Input: part model. Units: mm. Frame: model coordinates. Round coordinates to 2 decimals unless told otherwise and drop trailing zeros. Loops run counter-clockwise (first coordinate to the right, second up) from the corner with the lowest first, then second, coordinate; pieces in that order, holes last. Notation, with made-up numbers: M -10,76 L 47,76 A16 ccw 47,89 Z; hole C 18,52 d3. An arc over 180 degrees is marked long. Use one line per item in the form item = value. Start each with the question number.
Q1. Section query C-C, the plane y = 0. State how many separate pieces and enclosed holes the cut face has, and give its area (3 significant figures).
Q2. Section query B-B, the plane z = 3. Output: boundary loops of the cut face in (x, y) (3 decimals), and give its area (3 significant figures).
Q3. Mould query, pull axis Z, two halves, no side actions, for faces 1 (the cylindrical face through (7.4, -0.04, 23.75)), 2 (the flat face through (0, 2.925, 0)), 3 (the cylindrical face through (-25.24, 0.04, -5.6)). Classes: pulls with the +Z half, pulls with the -Z half, needs draft (parallel to the pull), parting line crosses it, or undercut.
Q4. Section query A-A, the plane x = 15. Output: boundary loops of the cut face in (y, z) (3 decimals).
Q5. First-contact query: P1, Ø3, axis at y = 2, z = -5.5, coming from the +X side. Flat tip, straight axial feed; report the tip coordinate or a pass-through.
Q6. Ray query, line 1 along Z through (x, y) = (13, -0.15); line 2 along X through (y, z) = (0.25, 6); line 3 along X through (y, z) = (-2.4, -21). Return the intervals inside material, ascending.
```python
from build123d import *

# Parameters (mm, degrees)
SKETCH1_R           = 25.85370091
BOSS_EXTRUDE1_DEPTH = 2.925
CUT_EXTRUDE1_DEPTH  = 38.02769506


with BuildPart() as part:
    # Sketch1 → Boss-Extrude1 (new, symmetric)
    with BuildSketch(Plane(origin=(0, 0, 0), x_dir=(1, 0, 0), z_dir=(0, 1, 0))):
        with Locations(Location((0, 0, 0), (0, 0, 270))):
            Circle(SKETCH1_R)
    extrude(amount=BOSS_EXTRUDE1_DEPTH, both=True)

    # Sketch2 → Cut-Extrude1 (cut, through all)
    with BuildSketch(Plane.XZ.offset(2.925)):
        with BuildLine():
            ThreePointArc((22.019698731, -5.602620776), (21.872491194, -7.364247848), (23.634118266, -7.511455385))
            ThreePointArc((23.634118266, -7.511455385), (23.781325803, -5.749828313), (22.019698731, -5.602620776))
        make_face()
        with BuildLine():
            ThreePointArc((22.791373624, 3.631983723), (22.644166087, 1.87035665), (24.405793159, 1.723149114))
            ThreePointArc((24.405793159, 1.723149114), (24.553000696, 3.484776186), (22.791373624, 3.631983723))
        make_face()
        with BuildLine():
            ThreePointArc((17.772833946, -13.838975667), (17.625626409, -15.600602739), (19.387253481, -15.747810276))
            ThreePointArc((19.387253481, -15.747810276), (19.534461018, -13.986183203), (17.772833946, -13.838975667))
        make_face()
        with BuildLine():
            ThreePointArc((10.697325934, -19.82317058), (10.550118397, -21.584797652), (12.311745469, -21.732005189))
            ThreePointArc((12.311745469, -21.732005189), (12.458953006, -19.970378117), (10.697325934, -19.82317058))
        make_face()
        with BuildLine():
            ThreePointArc((1.87035665, -22.644166087), (1.723149114, -24.405793159), (3.484776186, -24.553000696))
            ThreePointArc((3.484776186, -24.553000696), (3.631983723, -22.791373624), (1.87035665, -22.644166087))
        make_face()
        with BuildLine():
            ThreePointArc((-7.364247848, -21.872491194), (-7.511455385, -23.634118266), (-5.749828313, -23.781325803))
            ThreePointArc((-5.749828313, -23.781325803), (-5.602620776, -22.019698731), (-7.364247848, -21.872491194))
        make_face()
        with BuildLine():
            ThreePointArc((-15.600602739, -17.625626409), (-15.747810276, -19.387253481), (-13.986183203, -19.534461018))
            ThreePointArc((-13.986183203, -19.534461018), (-13.838975667, -17.772833946), (-15.600602739, -17.625626409))
        make_face()
        with BuildLine():
            ThreePointArc((-21.584797652, -10.550118397), (-21.732005189, -12.311745469), (-19.970378117, -12.458953006))
            ThreePointArc((-19.970378117, -12.458953006), (-19.82317058, -10.697325934), (-21.584797652, -10.550118397))
        make_face()
        with BuildLine():
            ThreePointArc((-24.405793159, -1.723149114), (-24.553000696, -3.484776186), (-22.791373624, -3.631983723))
            ThreePointArc((-22.791373624, -3.631983723), (-22.644166087, -1.87035665), (-24.405793159, -1.723149114))
        make_face()
        with BuildLine():
            ThreePointArc((-23.634118266, 7.511455385), (-23.781325803, 5.749828313), (-22.019698731, 5.602620776))
            ThreePointArc((-22.019698731, 5.602620776), (-21.872491194, 7.364247848), (-23.634118266, 7.511455385))
        make_face()
        with BuildLine():
            ThreePointArc((-19.387253481, 15.747810276), (-19.534461018, 13.986183203), (-17.772833946, 13.838975667))
            ThreePointArc((-17.772833946, 13.838975667), (-17.625626409, 15.600602739), (-19.387253481, 15.747810276))
        make_face()
        with BuildLine():
            ThreePointArc((-12.311745469, 21.732005189), (-12.458953006, 19.970378117), (-10.697325934, 19.82317058))
            ThreePointArc((-10.697325934, 19.82317058), (-10.550118397, 21.584797652), (-12.311745469, 21.732005189))
        make_face()
        with BuildLine():
            ThreePointArc((-3.484776186, 24.553000696), (-3.631983723, 22.791373624), (-1.87035665, 22.644166087))
            ThreePointArc((-1.87035665, 22.644166087), (-1.723149114, 24.405793159), (-3.484776186, 24.553000696))
        make_face()
        with BuildLine():
            ThreePointArc((5.749828313, 23.781325803), (5.602620776, 22.019698731), (7.364247848, 21.872491194))
            ThreePointArc((7.364247848, 21.872491194), (7.511455385, 23.634118266), (5.749828313, 23.781325803))
        make_face()
        with BuildLine():
            ThreePointArc((19.970378117, 12.458953006), (19.82317058, 10.697325934), (21.584797652, 10.550118397))
            ThreePointArc((21.584797652, 10.550118397), (21.732005189, 12.311745469), (19.970378117, 12.458953006))
        make_face()
        with BuildLine():
            ThreePointArc((13.986183203, 19.534461018), (13.838975667, 17.772833946), (15.600602739, 17.625626409))
            ThreePointArc((15.600602739, 17.625626409), (15.747810276, 19.387253481), (13.986183203, 19.534461018))
        make_face()
    extrude(amount=-CUT_EXTRUDE1_DEPTH, mode=Mode.SUBTRACT)


solid = part.part
```
Results found:
q1.separate_pieces = 1
q1.enclosed_holes = 16
q1.area = 2,020 mm²
q2.outline = M -25.679,-2.925 L 22.391,-2.925 L 22.391,2.925 L -25.679,2.925 Z; M 24.806,-2.925 L 25.679,-2.925 L 25.679,2.925 L 24.806,2.925 Z
q2.area = 286 mm²
q3.face_1 = undercut
q3.face_2 = needs draft
q3.face_3 = parting line crosses it
q4.outline = M -2.925,-21.057 L 2.925,-21.057 L 2.925,17.347 L -2.925,17.347 Z; M -2.925,19.813 L 2.925,19.813 L 2.925,21.057 L -2.925,21.057 Z
q5.P1 = 25.54
q6.line_1 = -22.35 to 22.35
q6.line_2 = -25.15 to -23.95, -21.71 to 25.15
q6.line_3 = -15.08 to 10.27, 12.73 to 15.08
